```python
from build123d import *

# Parameters (mm, degrees)
SKETCH22_W          = 159
SKETCH22_H          = 90
SKETCH22_R          = 4
SKETCH22_R_2        = 6.5
SKETCH22_W_2        = 99.6
SKETCH22_H_2        = 41
BOSS_EXTRUDE1_DEPTH = 3.15
BOSS_EXTRUDE2_DEPTH = 159
SKETCH25_R          = 1.25
CUT_EXTRUDE1_DEPTH  = 47.65
SKETCH26_R          = 1.5
CUT_EXTRUDE2_DEPTH  = 101.65
SKETCH28_R          = 3.175
SKETCH28_R_2        = 1
CUT_EXTRUDE3_DEPTH  = 47.65


with BuildPart() as part:
    # Sketch22 → Boss-Extrude1 (new body)
    with BuildSketch(Plane.XY):
        with Locations((-61.4, -14.5)):
            Rectangle(SKETCH22_W, SKETCH22_H)
        with Locations((0, -19.5)):
            Circle(SKETCH22_R, mode=Mode.SUBTRACT)
        with Locations((0, -36.5)):
            Circle(SKETCH22_R, mode=Mode.SUBTRACT)
        Circle(SKETCH22_R_2, mode=Mode.SUBTRACT)
        with Locations((-74.2, -23.3)):
            Rectangle(SKETCH22_W_2, SKETCH22_H_2, mode=Mode.SUBTRACT)
    extrude(amount=BOSS_EXTRUDE1_DEPTH)

    # Sketch23 → Boss-Extrude2 (add)
    with BuildSketch(Plane.ZY.offset(140.9)):
        with BuildLine():
            Line((0, -59.5), (3.15, -59.5))
            Line((3.15, -59.5), (3.15, -64))
            ThreePointArc((3.15, -64), (1.348706704, -68.348706704), (-3, -70.15))
            Line((-3, -70.15), (-43.5, -70.15))
            Line((-43.5, -70.15), (-43.5, -67))
            Line((-43.5, -67), (-3, -67))
            ThreePointArc((-3, -67), (-0.878679656, -66.121320344), (0, -64))
            Line((0, -64), (0, -59.5))
        make_face()
    extrude(amount=-BOSS_EXTRUDE2_DEPTH)

    # Sketch25 → Cut-Extrude1 (cut, through all)
    with BuildSketch(Plane.XY.offset(3.15)):
        with Locations((-133.8, 15.7)):
            Circle(SKETCH25_R)
        with Locations((11, 15.7)):
            Circle(SKETCH25_R)
    extrude(amount=-CUT_EXTRUDE1_DEPTH, mode=Mode.SUBTRACT)

    # Sketch26 → Cut-Extrude2 (cut, through all)
    with BuildSketch(Plane.XZ.offset(70.15)):
        with Locations((-133.8, -13)):
            Circle(SKETCH26_R)
        with Locations((11, -13)):
            Circle(SKETCH26_R)
    extrude(amount=-CUT_EXTRUDE2_DEPTH, mode=Mode.SUBTRACT)

    # Sketch28 → Cut-Extrude3 (cut, through all)
    with BuildSketch(Plane.XY.offset(3.15)):
        with Locations((-20, 16.5)):
            Circle(SKETCH28_R)
        with Locations((-13.9, 16.5)):
            Circle(SKETCH28_R_2)
    extrude(amount=-CUT_EXTRUDE3_DEPTH, mode=Mode.SUBTRACT)


solid = part.part
```
Here's how the part is built. I have some questions about the finished solid (model axes, mm). A direction names the side the tool comes from. Round coordinates to 2 decimals unless told otherwise and drop trailing zeros. Write each loop counter-clockwise with the first axis right and the second up, starting at its lowest first coordinate (ties: lowest second). Pieces come first, ordered by that corner, then holes.
Q1. If we section it at C-C on x = -126.5: Write out the boundary of the cut face in (y, z).
Q2. If we section it at B-B on x = -20: Write out the boundary of the cut face in (y, z) (3 decimals), plus the area to 3 significant figures.
Q3. If we section it at D-D on z = -32: Write out the boundary of the cut face in (x, y), plus the area to 3 significant figures.
Q4. Which directions (+Z, -Z, +X, -X, +Y, -Y) give clear straight access to the entire face, cutting with the end or side of a thin tool? Please do faces 5 (the flat face through (-24.4, -24, 2)), 6 (the flat face through (-63, -67, -24)), 7 (the flat face through (-63, -69, -43.5)).
Q5. If we section it at A-A on y = -19.5: Write out the boundary of the cut face in (x, z), plus the area to 3 significant figures.
Q6. Please list where these lines run through material, in increasing order: probe 1 along Y at (x, z) = (0, 2); probe 2 along Y at (x, z) = (-2.5, -23); probe 3 along Z at (x, y) = (-50, -63.5).
Q7. Will these pins go through, and if not, where does the flat tip stop? P1, Ø1.5, axis at x = -66.5, z = -25.5, coming from the +Y side; P2, Ø3.5, axis at x = -54.5, z = 2, coming from the -Y side; P3, Ø15, axis at x = 0, y = 0, coming from the -Z side.
Q8. If we mould it in two halves opening along Y, with no side actions, what happens to faces 1 (the flat face through (-63, 30.5, 2)), 2 (the flat face through (-63, 5, 3.15)), 3 (the cylindrical face through (-23.17, 16.64, 1.6)), 4 (the cylindrical face through (-5.158, -3.955, 1.553))? For each: +Y half, -Y half, draft (parallel to the pull), parting line (faces both ways), or undercut.
Answer below:
1. outline: (-70.15, -43.5) - (-67, -43.5) - (-67, -3) arc R3 cw to (-64, 0) - (30.5, 0) - (30.5, 3.15) - (-64, 3.15) arc R6.15 ccw to (-70.15, -3) - close
2. outline: (-70.15, -43.5) - (-67, -43.5) - (-67, -3) arc R3 cw to (-64, 0) - (13.325, 0) - (13.325, 3.15) - (-64, 3.15) arc R6.15 ccw to (-70.15, -3) - close; (19.675, 0) - (30.5, 0) - (30.5, 3.15) - (19.675, 3.15) - close
2. area: 428 mm2
3. outline: (-140.9, -70.15) - (18.1, -70.15) - (18.1, -67) - (-140.9, -67) - close
3. area: 501 mm2
4. face 5: +Z, -Z
4. face 6: -Z, +X, -X, +Y
4. face 7: -Z, +X, -X, +Y, -Y
5. outline: (-140.9, 0) - (-124, 0) - (-124, 3.15) - (-140.9, 3.15) - close; (-24.4, 0) - (-4, 0) - (-4, 3.15) - (-24.4, 3.15) - close; (4, 0) - (18.1, 0) - (18.1, 3.15) - (4, 3.15) - close
5. area: 162 mm2
6. probe 1: y = -67.58 to -40.5, -32.5 to -23.5, -15.5 to -6.5, 6.5 to 30.5
6. probe 2: y = -70.15 to -67
6. probe 3: z = 0 to 3.15
7. P1: stops at y = -67
7. P2: stops at y = -69.22
7. P3: stops at z = 0
8. face 1: +Y half
8. face 2: draft
8. face 3: undercut
8. face 4: undercut
